Could you check a few things on this model? Use its own coordinates, in mm. A direction names the side the tool comes from. Give positions to 0.01 mm unless a question says otherwise; leave off trailing zeros. Order: outer loops, then holes, each group sorted by start corner. A loop starts at its lowest first (then second) coordinate and runs counter-clockwise, first axis right, second up. Notation, with made-up numbers: (45.25, 44.5) -> (82.25, 44.5) arc R19 cw to (82.25, 68.5) -> close; hole circle Ø6 at (34, -21). An arc over 180 degrees is marked (long way). Write each question's results on one line, items separated by ' | '.
```python
from build123d import *

# Parameters (mm, degrees)
F1_DEPTH = 1000
F2_R     = 24.15
F3_DEPTH = 41.301


with BuildPart() as f1:
    # F0 (on Right) → F1 (new body)
    with BuildSketch(Plane.YZ):
        with BuildLine():
            Line((0, 38.8), (0, 2.5))
            ThreePointArc((0, 2.5), (0.732233, 0.732233), (2.5, 0))
            Line((2.5, 0), (7.05, 0))
            ThreePointArc((7.05, 0), (8.817767, 0.732233), (9.55, 2.5))
            Line((9.55, 2.5), (9.55, 3))
            Line((9.55, 3), (9.55, 6.5))
            ThreePointArc((9.55, 6.5), (9.403553, 6.853553), (9.05, 7))
            Line((9.05, 7), (7.05, 7))
            ThreePointArc((7.05, 7), (6.696447, 6.853553), (6.55, 6.5))
            Line((6.55, 6.5), (6.55, 3))
            Line((6.55, 3), (3, 3))
            Line((3, 3), (3, 38.3))
            Line((3, 38.3), (38.3, 38.3))
            Line((38.3, 38.3), (38.3, 3))
            Line((38.3, 3), (34.75, 3))
            Line((34.75, 3), (34.75, 6.5))
            ThreePointArc((34.75, 6.5), (34.603553, 6.853553), (34.25, 7))
            Line((34.25, 7), (32.25, 7))
            ThreePointArc((32.25, 7), (31.896447, 6.853553), (31.75, 6.5))
            Line((31.75, 6.5), (31.75, 3))
            Line((31.75, 3), (31.75, 2.5))
            ThreePointArc((31.75, 2.5), (32.482233, 0.732233), (34.25, 0))
            Line((34.25, 0), (38.8, 0))
            ThreePointArc((38.8, 0), (40.567767, 0.732233), (41.3, 2.5))
            Line((41.3, 2.5), (41.3, 38.8))
            ThreePointArc((41.3, 38.8), (40.567767, 40.567767), (38.8, 41.3))
            Line((38.8, 41.3), (2.5, 41.3))
            ThreePointArc((2.5, 41.3), (0.732233, 40.567767), (0, 38.8))
        make_face()
    extrude(amount=F1_DEPTH)

    # F2 (on face) → F3 (cut, through all)
    with BuildSketch(Plane.XY.offset(41.3)):
        with Locations((0, 20.65)):
            Circle(F2_R)
    extrude(amount=-F3_DEPTH, mode=Mode.SUBTRACT)


solid = f1.part
```
Q1. Suppose I cut it at B-B on x = 880.5. Please give me the cut outline in (y, z), and give its area (3 significant figures).
Here are the results:
outline: (0, 2.5) arc R2.5 ccw to (2.5, 0) -> (7.05, 0) arc R2.5 ccw to (9.55, 2.5) -> (9.55, 6.5) arc R0.5 ccw to (9.05, 7) -> (7.05, 7) arc R0.5 ccw to (6.55, 6.5) -> (6.55, 3) -> (3, 3) -> (3, 38.3) -> (38.3, 38.3) -> (38.3, 3) -> (34.75, 3) -> (34.75, 6.5) arc R0.5 ccw to (34.25, 7) -> (32.25, 7) arc R0.5 ccw to (31.75, 6.5) -> (31.75, 2.5) arc R2.5 ccw to (34.25, 0) -> (38.8, 0) arc R2.5 ccw to (41.3, 2.5) -> (41.3, 38.8) arc R2.5 ccw to (38.8, 41.3) -> (2.5, 41.3) arc R2.5 ccw to (0, 38.8) -> close | area: 409 mm²
Q2. I need wall thicknesses on line 1 along Y through (x, z) = (78.5, 37); line 2 along Z through (x, y) = (897, 34). Which ranges of each line are inside material? Lowest first, please.
Here are the results:
line 1: y = 0 to 3, 38.3 to 41.3 | line 2: z = 0.01 to 7, 38.3 to 41.3
Q3. Suppose I cut it at A-A on z = 18.5. Please give me the cut outline in (x, y), and give its area (3 significant figures).
Here are the results:
outline: (12.52, 0) -> (1000, 0) -> (1000, 3) -> (16.48, 3) arc R24.15 cw to start; (12.52, 41.3) arc R24.15 cw to (16.48, 38.3) -> (1000, 38.3) -> (1000, 41.3) -> close | area: 5,910 mm²
Q4. Suppose I cut it at C-C on y = 21.5. Please give me the cut outline in (x, z), and give its area (3 significant figures).
Here are the results:
outline: (24.14, 38.3) -> (1000, 38.3) -> (1000, 41.3) -> (24.14, 41.3) -> close | area: 2,930 mm²
Q5. For faces 1 (the flat face through (1000, 21, 39)), 2 (the flat face through (501, 20, 38.3)), which set-ups out of +Z, -Z, +X, -X, +Y, -Y let a thin tool reach every point of the face, with its end or its side?
Here are the results:
face 1: +Z, -Z, +X, +Y, -Y | face 2: +X, -X
Q6. Thinking about a two-plate mould opening in Y: for faces 3 (the flat face through (501, 21, 41.3)), 4 (the flat face through (501, 38.3, 21)), 5 (the flat face through (499, 0, 21)), which applies, +Y half, -Y half, draft (parallel to the pull), parting line (faces both ways), or undercut?
Here are the results:
face 3: draft | face 4: undercut | face 5: -Y half
